For this review, take the finished solid that the model builds, in its own axes (mm). Face numbers are marked on the shaded views. A direction names the side the tool comes from. Round coordinates to 2 decimals unless told otherwise and drop trailing zeros. Order: outer loops, then holes, each group sorted by start corner. A loop starts at its lowest first (then second) coordinate and runs counter-clockwise, first axis right, second up. Notation, with made-up numbers: M 37.25,-27.5 L 53.25,-27.5 A29 cw 53.25,6.5 Z; hole C 16.5,2.25 d7. An arc over 180 degrees is marked long. Use a Markdown table: item, result.
from build123d import *

# Parameters (mm, degrees)
SKETCH1_W           = 92.3
SKETCH1_H           = 30.5
SKETCH1_W_2         = 84.3
SKETCH1_H_2         = 26.5
BOSS_EXTRUDE1_DEPTH = 3
SKETCH2_W           = 3
SKETCH2_H           = 3
BOSS_EXTRUDE2_DEPTH = 5
SKETCH13_W          = 92.3
SKETCH13_H          = 30.5
SKETCH13_W_2        = 83.8
SKETCH13_H_2        = 26
CUT_EXTRUDE9_DEPTH  = 5
SKETCH12_R          = 1.25
CUT_EXTRUDE8_DEPTH  = 12
BOSS_EXTRUDE4_DEPTH = 30.5
FILLET1_R           = 4
SKETCH15_R          = 4.5
CUT_EXTRUDE10_DEPTH = 51


with BuildPart() as part:
    # Sketch1 → Boss-Extrude1 (new body)
    # profile 1 of 2: a face of its own
    with BuildSketch(Plane.XY):
        with Locations((0, 0.6)):
            Rectangle(SKETCH1_W, SKETCH1_H)
        with Locations((0, 0.6)):
            Rectangle(SKETCH1_W_2, SKETCH1_H_2, mode=Mode.SUBTRACT)
    # profile 2 of 2: a face of its own
    with BuildSketch(Plane.XY):
        with Locations((0, 0.6)):
            Rectangle(SKETCH1_W_2, SKETCH1_H_2)
    extrude(amount=BOSS_EXTRUDE1_DEPTH)

    # Sketch2 → Boss-Extrude2 (add)
    with BuildSketch(Plane.XY.offset(3)):
        with Locations((-40.65, 12.35)):
            Rectangle(SKETCH2_W, SKETCH2_H)
        with Locations((40.65, 12.35)):
            Rectangle(SKETCH2_W, SKETCH2_H)
        with Locations((40.65, -11.15)):
            Rectangle(SKETCH2_W, SKETCH2_H)
        with Locations((-40.65, -11.15)):
            Rectangle(SKETCH2_W, SKETCH2_H)
    extrude(amount=BOSS_EXTRUDE2_DEPTH)

    # Sketch13 → Cut-Extrude9 (cut)
    with BuildSketch(Plane.XY.offset(8)):
        with Locations((0, 0.6)):
            Rectangle(SKETCH13_W, SKETCH13_H)
        with Locations((0, 0.6)):
            Rectangle(SKETCH13_W_2, SKETCH13_H_2, mode=Mode.SUBTRACT)
    extrude(amount=-CUT_EXTRUDE9_DEPTH, mode=Mode.SUBTRACT)

    # Sketch12 → Cut-Extrude8 (cut)
    with BuildSketch(Plane.XY.offset(3)):
        with Locations((-28.15, -7.15)):
            Circle(SKETCH12_R)
    extrude(amount=-CUT_EXTRUDE8_DEPTH, mode=Mode.SUBTRACT)

    # Sketch14 → Boss-Extrude4 (add)
    with BuildSketch(Plane(origin=(0, 15.85, 0), x_dir=(1, 0, 0), z_dir=(0, 1, 0))):
        with BuildLine():
            Line((12.799828546, 44.630563997), (13.151366909, 14.632623721))
            Line((13.151366909, 14.632623721), (19.974671409, 0))
            Line((19.974671409, 0), (24.687430993, 0))
            Line((24.687430993, 0), (18.887905283, 12.437123022))
            ThreePointArc((18.887905283, 12.437123022), (18.338278668, 14.040820406), (18.138916839, 15.724325552))
            Line((18.138916839, 15.724325552), (17.823136491, 42.670915272))
            ThreePointArc((17.823136491, 42.670915272), (17.22518506, 44.073889153), (15.812063723, 44.647447965))
            Line((15.812063723, 44.647447965), (12.799828546, 44.630563997))
        make_face()
        with BuildLine():
            Line((-13.151397234, 14.632558688), (-12.798784772, 44.487080457))
            Line((-12.798784772, 44.487080457), (-15.83402069, 44.470067567))
            ThreePointArc((-15.83402069, 44.470067567), (-17.23263166, 43.888691454), (-17.822671194, 42.493713254))
            Line((-17.822671194, 42.493713254), (-18.138767444, 15.72395041))
            ThreePointArc((-18.138767444, 15.72395041), (-18.338200149, 14.040810917), (-18.887747495, 12.4374614))
            Line((-18.887747495, 12.4374614), (-24.687430993, 0))
            Line((-24.687430993, 0), (-19.974671409, 0))
            Line((-19.974671409, 0), (-13.151397234, 14.632558688))
        make_face()
    extrude(amount=-BOSS_EXTRUDE4_DEPTH)

    # Fillet1
    fillet1_edges = [part.edges().sort_by_distance(p)[0] for p in [
        (24.687430993, 0.6, 0),
        (19.974671409, 0.6, 0),
        (-19.974671409, 0.6, 0),
        (-24.687430993, 0.6, 0),
    ]]
    fillet(fillet1_edges, radius=FILLET1_R)

    # Sketch15 → Cut-Extrude10 (cut)
    with BuildSketch(Plane(origin=(-18.321880618, 0, -0.216344007), x_dir=(-0.011807135462763681, 0, 0.9999302933465732), z_dir=(-0.9999302933465732, 0, -0.011807135462763681))):
        with Locations((-34.28001328, 0.6)):
            Circle(SKETCH15_R)
        with BuildLine():
            Line((-39.121242463, 15.85), (-39.121242463, 17.869989606))
            Line((-39.121242463, 17.869989606), (-55.967413811, 17.869989606))
            Line((-55.967413811, 17.869989606), (-55.967413811, -17.820804899))
            Line((-55.967413811, -17.820804899), (-39.121242463, -17.820804899))
            Line((-39.121242463, -17.820804899), (-39.121242463, -14.65))
            ThreePointArc((-39.121242463, -14.65), (-50.28001328, 0.6), (-39.121242463, 15.85))
        make_face()
        with BuildLine():
            Line((-36.156004252, -6.661587834), (-36.90640064, -9.566222968))
            ThreePointArc((-36.90640064, -9.566222968), (-27.850669118, -7.701417568), (-23.78001328, 0.6))
            Line((-23.78001328, 0.6), (-26.78001328, 0.6))
            ThreePointArc((-26.78001328, 0.6), (-29.687624593, -5.329583977), (-36.156004252, -6.661587834))
        make_face()
    extrude(amount=-CUT_EXTRUDE10_DEPTH, mode=Mode.SUBTRACT)


solid = part.part
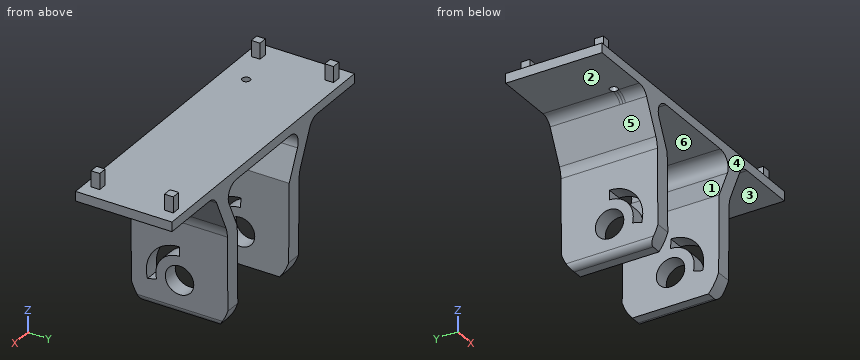
Q1. Draft analysis for pull direction X (two halves, no side actions). For the marked faces 4, 5 and 6, state which applies: pulls with the +X half, pulls with the -X half, needs draft (parallel to the pull), parting line crosses it, or undercut.
Determined:
| item | result |
|---|---|
| face 4 | needs draft |
| face 5 | pulls with the -X half |
| face 6 | undercut |
Q2. Add section A-A (x = -28.15). Write out the cut boundary in (y, z).
Determined:
| item | result |
|---|---|
| outline | M -14.65,0 L -8.4,0 L -8.4,3 L -14.65,3 Z; M -5.9,0 L 15.85,0 L 15.85,3 L -5.9,3 Z |
Q3. Add section C-C (z = -4). Write out the cut boundary in (x, y).
Determined:
| item | result |
|---|---|
| outline | M -22.82,-14.65 L -17.7,-14.65 L -17.7,15.85 L -22.82,15.85 Z; M 17.7,-14.65 L 22.82,-14.65 L 22.82,15.85 L 17.7,15.85 Z |
Q4. Wall thickness on line 1 along X through (y, z) = (-7, 1); line 2 along Y through (x, z) = (-28.15, 0.8); line 3 along Z through (x, y) = (-13.5, -8): over which ranges is each line inside the solid? List them lowest first. Write a range as [from, to].
Determined:
| item | result |
|---|---|
| line 1 | x = [-46.15, -29.39], [-26.91, 46.15] |
| line 2 | y = [-14.65, -8.4], [-5.9, 15.85] |
| line 3 | z = [-44.48, -36.66], [-28.42, -13.88], [0, 3] |
Q5. Clearance check with flat-ended pins moving along their axes: pin 1 (0.8 mm diameter, centred on x = -40.5, z = 6.5, fed in from +Y); pin 2 (10 mm diameter, centred on x = -19.5, y = -1, fed in from -Z); pin 3 (1.4 mm diameter, centred on x = 40, z = 4.5, fed in from -Y); pin 4 (5 mm diameter, centred on x = -21.5, z = -11, fed in from +Y). State where each tip first meets the part, or that it passes through.
Determined:
| item | result |
|---|---|
| pin 1 | stops at y = 13.6 |
| pin 2 | stops at z = -44.48 |
| pin 3 | stops at y = -12.4 |
| pin 4 | stops at y = 15.85 |
Q6. Add section B-B (y = 2.5). Give the number of separate pieces and of enclosed holes in the cut face, then the cut area to 3 significant figures.
Determined:
| item | result |
|---|---|
| separate pieces | 3 |
| enclosed holes | 0 |
| area | 652 mm^2 |
Q7. Add section D-D (x = 40.5). Write out the cut boundary in (y, z).
Determined:
| item | result |
|---|---|
| outline | M -14.65,0 L 15.85,0 L 15.85,3 L 13.6,3 L 13.6,8 L 10.85,8 L 10.85,3 L -9.65,3 L -9.65,8 L -12.4,8 L -12.4,3 L -14.65,3 Z |
Q8. Machinability: for the marked faces 1, 2 and 3, which of the approach directions +Z, -Z, +X, -X, +Y, -Y give a long, thin tool a straight path to every point of the face, cutting with its end or side? Answer none if there is none.
Determined:
| item | result |
|---|---|
| face 1 | +Y, -Y |
| face 2 | -Z, -X, +Y, -Y |
| face 3 | -Z, +X, +Y, -Y |
